Check sheet for the modelled part. Datum: model origin and axes. Units: mm. Face numbers are marked on the shaded views. A direction names the side the tool comes from. Coordinates: 2 decimals unless noted, no trailing zeros. Order: outer loops, then holes, each group sorted by start corner. A loop starts at its lowest first (then second) coordinate and runs counter-clockwise, first axis right, second up.
from build123d import *

# Parameters (mm, degrees)
F0_W     = 47
F0_H     = 2
F0_W_2   = 10
F0_H_2   = 3.4
F1_DEPTH = 4
F2_DEPTH = 10
F3_R     = 1


with BuildPart() as f1:
    # F0 (on Top) → F1 (new body)
    with BuildSketch(Plane.XY):
        with Locations((-12.59553, 9.557682)):
            Rectangle(F0_W, F0_H)
        Polygon((10.90447, 10.657682), (10.90447, 10.557682), (10.90447, 8.557682), (10.90447, 3.057682), (32.90447, 3.057682), (32.90447, 14.057682), (20.90447, 14.057682), (20.90447, 10.657682), align=None)
        with Locations((15.90447, 12.357682)):
            Rectangle(F0_W_2, F0_H_2)
    extrude(amount=F1_DEPTH)

    # F0 (on Top) → F2 (join)
    with BuildSketch(Plane.XY):
        with Locations((15.90447, 12.357682)):
            Rectangle(F0_W_2, F0_H_2)
    extrude(amount=-F2_DEPTH)

    # F3
    f3_edges = [f1.edges().sort_by_distance(p)[0] for p in [
        (32.90447, 3.057682, 2),
        (32.90447, 14.057682, 2),
    ]]
    fillet(f3_edges, radius=F3_R)


solid = f1.part
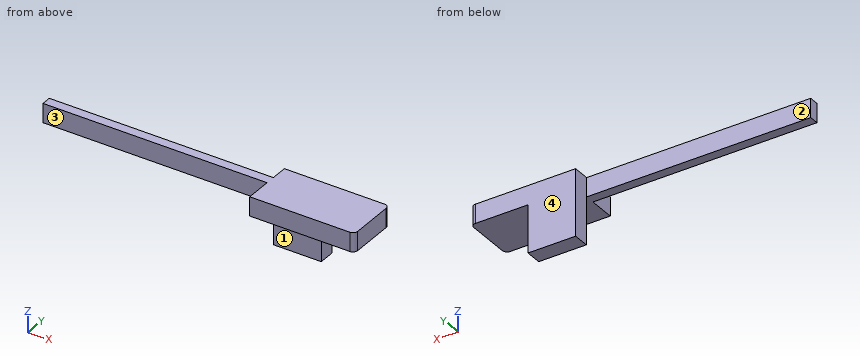
(1) Tool access check on the marked faces 1, 2, 3 and 4. Record the directions out of +Z, -Z, +X, -X, +Y, -Y that give a thin tool (end or side, any length) a straight path to the whole face; none if there is none.
Filled in:
face 1: -Z, +X, -X, -Y
face 2: +Z, -Z, -X, +Y
face 3: +Z, -Z, -X, -Y
face 4: +Z, -Z, +X, -X, +Y
(2) Cross-section at C-C (x = -6). Enter the section's corners in (y, z).
Filled in:
outline: (8.56, 0) - (10.56, 0) - (10.56, 4) - (8.56, 4) - close
(3) Go/stop test with flat-tipped pins: P1, Ø5.5, axis at x = -15, y = 11, coming from the -Z side; P2, Ø2, axis at y = 7, z = 2, coming from the -X side; P3, Ø1.2, axis at x = -2.5, z = 3, coming from the +Y side. Record where each tip stops, or that it passes through.
Filled in:
P1: stops at z = 0
P2: stops at x = 10.9
P3: stops at y = 10.56
(4) Cross-section at A-A (y = 12). Enter the section's corners in (x, z).
Filled in:
outline: (10.9, -10) - (20.9, -10) - (20.9, 0) - (32.9, 0) - (32.9, 4) - (10.9, 4) - close
(5) Thickness scan on probe 1 along X at (y, z) = (6.25, 2.25); probe 2 along X at (y, z) = (11.5, -2.75); probe 3 along Z at (x, y) = (30, 6.5). Record the ranges inside material, lowest first.
Filled in:
probe 1: x = 10.9 to 32.9
probe 2: x = 10.9 to 20.9
probe 3: z = 0 to 4
(6) Cross-section at B-B (z = 2.5). Enter the section's corners in (x, y).
Filled in:
outline: (-36.1, 8.56) - (10.9, 8.56) - (10.9, 3.06) - (31.9, 3.06) arc R1 ccw to (32.9, 4.06) - (32.9, 13.06) arc R1 ccw to (31.9, 14.06) - (10.9, 14.06) - (10.9, 10.56) - (-36.1, 10.56) - close
(7) Cross-section at D-D (z = -8). Enter the section's corners in (x, y), and give its area (3 significant figures).
Filled in:
outline: (10.9, 10.66) - (20.9, 10.66) - (20.9, 14.06) - (10.9, 14.06) - close
area: 34.0 mm2
